Build history of the part. All positions in model axes, mm. Coordinates: 2 decimals unless noted, no trailing zeros. Write each loop counter-clockwise with the first axis right and the second up, starting at its lowest first coordinate (ties: lowest second). Pieces come first, ordered by that corner, then holes. Notation, with made-up numbers: (4.5, 23.5) -> (22.5, 23.5) arc R19 cw to (22.5, 30.5) -> close; hole circle Ø6 at (47, -28.75). An arc over 180 degrees is marked (long way). Write each question's results on one line, items separated by ' | '. Start each with the question number.
Q1. Saw through at A-A on y = 79. Give the cut face in (x, z).
Q2. Drop flat-ended pins along their axis: pin 1 Ø4 at (x, y) = (-7, 245.5) entering from +Z; pin 2 Ø1.5 at (x, z) = (7.5, -9) entering from -Y; pin 3 Ø10 at (y, z) = (301, -9) entering from -X. Give the stop position or say it passes through.
Q3. Drill centre lines: line 1 (X direction, y = 129, z = -1.25); line 2 (X direction, y = 935.5, z = -1.5); line 3 (Y direction, x = -0.5, z = 11). Where is each one in solid material? Low to high.
from build123d import *


with BuildPart() as f3:
    # F3: sweep along a path in F1
    with BuildLine(Plane.XZ) as f3_path:
        CenterArc((0, 0), 17.204414341, 0, 360)
    # F0 (on Right) → F3 (sweep)
    with BuildSketch(Plane.YZ):
        Polygon((-25.4, -6.35), (-25.4, -9.525), (38.1, -9.525), (38.1, -12.7), (482.6, -12.7), (482.6, 0), (-44.45, 0), (-44.45, -6.35), align=None)
    sweep(path=f3_path.line)

    # F4: F3 across plane


with BuildPart() as f3_1:
    add(f3.part)
    add(f3.part.mirror(Plane(origin=(0, 482.6, 0), x_dir=(-1, 0, 0), z_dir=(0, 1, 0))))


solid = f3_1.part
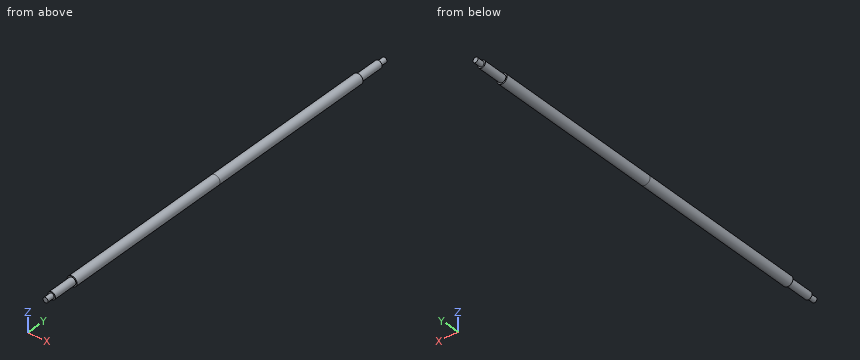
Returned:
1) outline: circle Ø25.4 at (0, 0)
2) pin 1: stops at z = 11.67 | pin 2: stops at y = 38.1 | pin 3: stops at x = -12.05
3) line 1: x = -12.64 to 12.64 | line 2: x = -9.41 to 9.41 | line 3: y = 38.1 to 927.1
